Verification items for this drawing (mm, ordinates from the low corner). Round coordinates to 2 decimals unless told otherwise and drop trailing zeros. Order: outer loops, then holes, each group sorted by start corner. A loop starts at its lowest first (then second) coordinate and runs counter-clockwise, first axis right, second up. Notation, with made-up numbers: (-38, 13.5) - (21, 13.5) arc R35 ccw to (21, 47.5) - close; hole circle Ø11 at (-23, 56). An arc over 180 degrees is marked (long way). Use a Markdown table: item, result. Add a question column.
(1) Thickness scan on line 1 along X through (y, z) = (1.7, 7) (3 decimals); line 2 along Z through (x, y) = (44.5, 1.65). Record the ranges inside material, lowest first. Write a range as [from, to].
(2) Gauge pin test, flat end, axial feed: P1, Ø1, axis at x = 46, y = 1.5, coming from the +Z side. Record the tip position at first contact, or that the pin passes through.
(3) Section check B-B on y = 1.9. Record the boundary of the cut face in (x, z) (3 decimals).
(4) Section check A-A on z = 9.25. Record the boundary of the cut face in (x, y) (3 decimals).
(5) Section check C-C on x = 61.5. Record the boundary of the cut face in (y, z) (3 decimals).
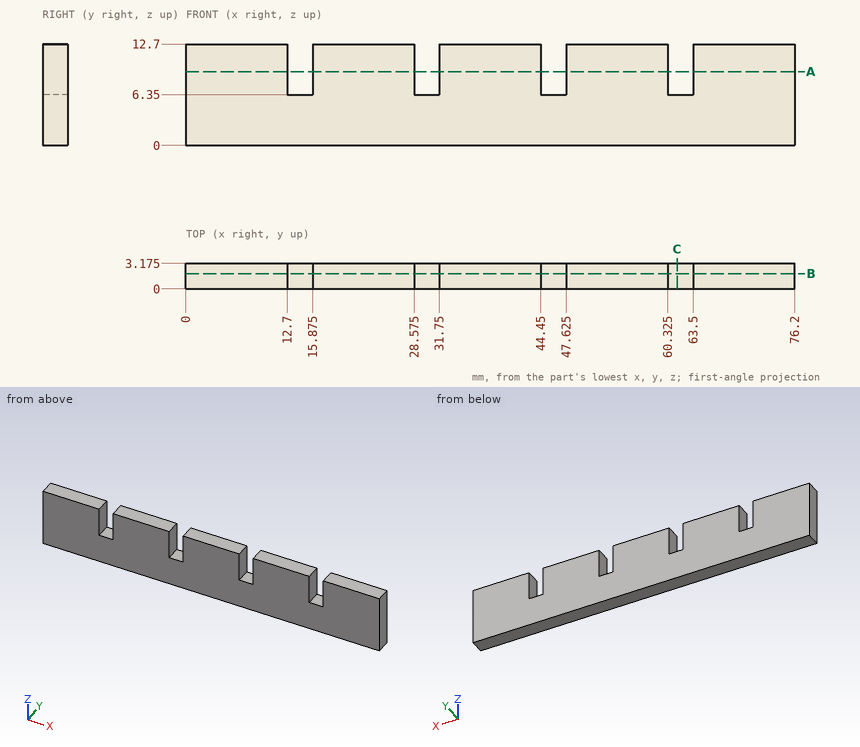
Check sheet entries:
| question | item | result |
|---|---|---|
| 1 | line 1 | x = [0, 12.7], [15.875, 28.575], [31.75, 44.45], [47.625, 60.325], [63.5, 76.2] |
| 1 | line 2 | z = [0, 6.35] |
| 2 | P1 | stops at z = 6.35 |
| 3 | outline | (0, 0) - (76.2, 0) - (76.2, 12.7) - (63.5, 12.7) - (63.5, 6.35) - (60.325, 6.35) - (60.325, 12.7) - (47.625, 12.7) - (47.625, 6.35) - (44.45, 6.35) - (44.45, 12.7) - (31.75, 12.7) - (31.75, 6.35) - (28.575, 6.35) - (28.575, 12.7) - (15.875, 12.7) - (15.875, 6.35) - (12.7, 6.35) - (12.7, 12.7) - (0, 12.7) - close |
| 4 | outline | (0, 0) - (12.7, 0) - (12.7, 3.175) - (0, 3.175) - close; (15.875, 0) - (28.575, 0) - (28.575, 3.175) - (15.875, 3.175) - close; (31.75, 0) - (44.45, 0) - (44.45, 3.175) - (31.75, 3.175) - close; (47.625, 0) - (60.325, 0) - (60.325, 3.175) - (47.625, 3.175) - close; (63.5, 0) - (76.2, 0) - (76.2, 3.175) - (63.5, 3.175) - close |
| 5 | outline | (0, 0) - (3.175, 0) - (3.175, 6.35) - (0, 6.35) - close |
